Input: part model. Units: mm. Frame: model coordinates. A direction names the side the tool comes from. Coordinates: 2 decimals unless noted, no trailing zeros. Loops run counter-clockwise (first coordinate to the right, second up) from the corner with the lowest first, then second, coordinate; pieces in that order, holes last. Notation, with made-up numbers: (43, 48) - (65, 48) arc R27 cw to (65, 74) - close; hole circle Ø3 at (25.25, -14.75). An arc over 180 degrees is marked (long way). Use a Markdown table: item, result. Add a question column.
1. Access query for faces 1 (the face through (21, -21, -30)), 2 (the face through (-1, -43, -26)). Directions: +Z, -Z, +X, -X, +Y, -Y. A direction counts if a zero-diameter tool reaches every point of the face in a straight line with its end or side. Return the directions, or none.
2. Ray query, L1, parallel to Y at x = 0, z = -11; L2, parallel to Z at x = -18.5, y = -59; L3, parallel to X at y = -22, z = 11. Return the intervals inside material, ascending. Write a range as [from, to].
3. Section query A-A on y = 0. Return the cut outline in (x, z), then the cut area to 3 significant figures.
4. Draft query along Y for faces 3 (the face through (-7.262, -32.703, -0.364)), 4 (the face through (14.246, 22.345, -0.42)), 5 (the face through (-1, -43, 26)). Return one class per face: released by +Y, released by -Y, zero draft, split by the parting line, or undercut.
5. Section query C-C on z = 16. Return the cut outline in (x, y), then the cut area to 3 significant figures.
6. Section query D-D on y = 80. Return the cut outline in (x, z).
7. Contact query for a flat-ended pin moving along its axis: P1, Ø4, axis at x = 10.5, z = 12.5, coming from the +Y side. Output: stop coordinate, or through.
```python
from build123d import *

# Parameters (mm, degrees)
SKETCH1_R           = 100
SKETCH1_R_2         = 26.5
BOSS_EXTRUDE1_DEPTH = 30
SKETCH2_R           = 100
SKETCH2_R_2         = 33.5
CUT_EXTRUDE1_DEPTH  = 26


with BuildPart() as part:
    # Sketch1 → Boss-Extrude1 (new body, symmetric)
    with BuildSketch(Plane.XY):
        Circle(SKETCH1_R)
        Circle(SKETCH1_R_2, mode=Mode.SUBTRACT)
    extrude(amount=BOSS_EXTRUDE1_DEPTH, both=True)

    # Sketch2 → Cut-Extrude1 (cut, symmetric)
    with BuildSketch(Plane.XY):
        Circle(SKETCH2_R)
        Circle(SKETCH2_R_2, mode=Mode.SUBTRACT)
    extrude(amount=CUT_EXTRUDE1_DEPTH, both=True, mode=Mode.SUBTRACT)


solid = part.part
```
Resolved:
| question | item | result |
|---|---|---|
| 1 | face 1 | -Z, +X, -X, +Y, -Y |
| 1 | face 2 | none |
| 2 | L1 | [-33.5, -26.5], [26.5, 33.5] |
| 2 | L2 | [-30, -26], [26, 30] |
| 2 | L3 | [-25.26, -14.77], [14.77, 25.26] |
| 3 | outline | (-100, -30) - (-26.5, -30) - (-26.5, 30) - (-100, 30) - (-100, 26) - (-33.5, 26) - (-33.5, -26) - (-100, -26) - close; (26.5, -30) - (100, -30) - (100, -26) - (33.5, -26) - (33.5, 26) - (100, 26) - (100, 30) - (26.5, 30) - close |
| 3 | area | 1,900 mm² |
| 4 | face 3 | split by the parting line |
| 4 | face 4 | undercut |
| 4 | face 5 | zero draft |
| 5 | outline | circle Ø67 at (0, 0); hole circle Ø53 at (0, 0) |
| 5 | area | 1,320 mm² |
| 6 | outline | (-60, -30) - (60, -30) - (60, -26) - (-60, -26) - close; (-60, 26) - (60, 26) - (60, 30) - (-60, 30) - close |
| 7 | P1 | y = 32.4 |
